Can you work these out from the model? Positions are in its coordinate system, mm. A direction names the side the tool comes from. Coordinates: 2 decimals unless noted, no trailing zeros. Order: outer loops, then holes, each group sorted by start corner. A loop starts at its lowest first (then second) coordinate and runs counter-clockwise, first axis right, second up.
```python
from build123d import *

# Parameters (mm, degrees)
SKETCH1_R           = 1.5
SKETCH1_R_2         = 3
BOSS_EXTRUDE1_DEPTH = 4
BOSS_EXTRUDE2_START = 4
SKETCH1_4_R         = 1.5
SKETCH1_4_R_2       = 3
BOSS_EXTRUDE2_DEPTH = 4
FILLET1_R           = 6
FILLET2_R           = 6
FILLET3_R           = 3
FILLET4_R           = 10


with BuildPart() as part:
    # Sketch1 → Boss-Extrude1 (new body)
    with BuildSketch(Plane(origin=(0, 0, 0), x_dir=(1, 0, 0), z_dir=(0, 1, 0))):
        Polygon((-84.75, 12.5), (-84.75, -12.5), (-67.174137787, -12.5), (-42.636751346, -55), (84.75, -55), (84.75, -45), (49.90212315, -45), (31.138239402, -12.5), (84.75, -12.5), (84.75, 12.5), (31.138239402, 12.5), (49.90212315, 45), (84.75, 45), (84.75, 55), (-42.636751346, 55), (-67.174137787, 12.5), align=None)
        Polygon((26.519437248, 12.5), (6.519437248, 12.5), (-12.244446501, 45), (45.283320997, 45), align=None, mode=Mode.SUBTRACT)
        Polygon((45.283320997, -45), (-12.244446501, -45), (6.519437248, -12.5), (26.519437248, -12.5), align=None, mode=Mode.SUBTRACT)
        Polygon((1.900635095, 12.5), (-55.627132403, 12.5), (-36.863248654, 45), (-16.863248654, 45), align=None, mode=Mode.SUBTRACT)
        Polygon((-16.863248654, -45), (-36.863248654, -45), (-55.627132403, -12.5), (1.900635095, -12.5), align=None, mode=Mode.SUBTRACT)
        with Locations(Location((-80.25, -7.5, 0), (0, 0, 270))):
            Circle(SKETCH1_R, mode=Mode.SUBTRACT)
        with Locations(Location((-65.25, -7.5, 0), (0, 0, 270))):
            Circle(SKETCH1_R, mode=Mode.SUBTRACT)
        with Locations(Location((-59.75, 0, 0), (0, 0, 270))):
            Circle(SKETCH1_R, mode=Mode.SUBTRACT)
        with Locations(Location((-49.75, 0, 0), (0, 0, 270))):
            Circle(SKETCH1_R, mode=Mode.SUBTRACT)
        with Locations(Location((-39.75, 0, 0), (0, 0, 270))):
            Circle(SKETCH1_R, mode=Mode.SUBTRACT)
        with Locations(Location((-29.75, 0, 0), (0, 0, 270))):
            Circle(SKETCH1_R, mode=Mode.SUBTRACT)
        with Locations(Location((-19.75, 0, 0), (0, 0, 270))):
            Circle(SKETCH1_R, mode=Mode.SUBTRACT)
        with Locations(Location((-9.75, 0, 0), (0, 0, 270))):
            Circle(SKETCH1_R, mode=Mode.SUBTRACT)
        with Locations(Location((0.25, 0, 0), (0, 0, 270))):
            Circle(SKETCH1_R, mode=Mode.SUBTRACT)
        with Locations(Location((10.25, 0, 0), (0, 0, 270))):
            Circle(SKETCH1_R, mode=Mode.SUBTRACT)
        with Locations(Location((20.25, 0, 0), (0, 0, 270))):
            Circle(SKETCH1_R, mode=Mode.SUBTRACT)
        with Locations(Location((30.25, 0, 0), (0, 0, 270))):
            Circle(SKETCH1_R, mode=Mode.SUBTRACT)
        with Locations(Location((40.25, 0, 0), (0, 0, 270))):
            Circle(SKETCH1_R, mode=Mode.SUBTRACT)
        with Locations(Location((50.25, 0, 0), (0, 0, 270))):
            Circle(SKETCH1_R, mode=Mode.SUBTRACT)
        with Locations(Location((-72.75, 0, 0), (0, 0, 270))):
            Circle(SKETCH1_R_2, mode=Mode.SUBTRACT)
        with Locations(Location((-80.25, 7.5, 0), (0, 0, 270))):
            Circle(SKETCH1_R, mode=Mode.SUBTRACT)
        with Locations(Location((-65.25, 7.5, 0), (0, 0, 270))):
            Circle(SKETCH1_R, mode=Mode.SUBTRACT)
        with Locations(Location((50.25, -50, 0), (0, 0, 270))):
            Circle(SKETCH1_R, mode=Mode.SUBTRACT)
        with Locations(Location((-39.75, -50, 0), (0, 0, 270))):
            Circle(SKETCH1_R, mode=Mode.SUBTRACT)
        with Locations(Location((-29.75, -50, 0), (0, 0, 270))):
            Circle(SKETCH1_R, mode=Mode.SUBTRACT)
        with Locations(Location((-19.75, -50, 0), (0, 0, 270))):
            Circle(SKETCH1_R, mode=Mode.SUBTRACT)
        with Locations(Location((-9.75, -50, 0), (0, 0, 270))):
            Circle(SKETCH1_R, mode=Mode.SUBTRACT)
        with Locations(Location((0.25, -50, 0), (0, 0, 270))):
            Circle(SKETCH1_R, mode=Mode.SUBTRACT)
        with Locations(Location((10.25, -50, 0), (0, 0, 270))):
            Circle(SKETCH1_R, mode=Mode.SUBTRACT)
        with Locations(Location((20.25, -50, 0), (0, 0, 270))):
            Circle(SKETCH1_R, mode=Mode.SUBTRACT)
        with Locations(Location((30.25, -50, 0), (0, 0, 270))):
            Circle(SKETCH1_R, mode=Mode.SUBTRACT)
        with Locations(Location((40.25, -50, 0), (0, 0, 270))):
            Circle(SKETCH1_R, mode=Mode.SUBTRACT)
        with Locations(Location((50.25, 50, 0), (0, 0, 270))):
            Circle(SKETCH1_R, mode=Mode.SUBTRACT)
        with Locations(Location((-39.75, 50, 0), (0, 0, 270))):
            Circle(SKETCH1_R, mode=Mode.SUBTRACT)
        with Locations(Location((-29.75, 50, 0), (0, 0, 270))):
            Circle(SKETCH1_R, mode=Mode.SUBTRACT)
        with Locations(Location((-19.75, 50, 0), (0, 0, 270))):
            Circle(SKETCH1_R, mode=Mode.SUBTRACT)
        with Locations(Location((-9.75, 50, 0), (0, 0, 270))):
            Circle(SKETCH1_R, mode=Mode.SUBTRACT)
        with Locations(Location((0.25, 50, 0), (0, 0, 270))):
            Circle(SKETCH1_R, mode=Mode.SUBTRACT)
        with Locations(Location((10.25, 50, 0), (0, 0, 270))):
            Circle(SKETCH1_R, mode=Mode.SUBTRACT)
        with Locations(Location((20.25, 50, 0), (0, 0, 270))):
            Circle(SKETCH1_R, mode=Mode.SUBTRACT)
        with Locations(Location((30.25, 50, 0), (0, 0, 270))):
            Circle(SKETCH1_R, mode=Mode.SUBTRACT)
        with Locations(Location((40.25, 50, 0), (0, 0, 270))):
            Circle(SKETCH1_R, mode=Mode.SUBTRACT)
        with Locations(Location((80.25, -50, 0), (0, 0, 270))):
            Circle(SKETCH1_R, mode=Mode.SUBTRACT)
        with Locations(Location((60.25, -50, 0), (0, 0, 270))):
            Circle(SKETCH1_R, mode=Mode.SUBTRACT)
        with Locations(Location((70.25, -50, 0), (0, 0, 270))):
            Circle(SKETCH1_R, mode=Mode.SUBTRACT)
        with Locations(Location((80.25, 50, 0), (0, 0, 270))):
            Circle(SKETCH1_R, mode=Mode.SUBTRACT)
        with Locations(Location((60.25, 50, 0), (0, 0, 270))):
            Circle(SKETCH1_R, mode=Mode.SUBTRACT)
        with Locations(Location((70.25, 50, 0), (0, 0, 270))):
            Circle(SKETCH1_R, mode=Mode.SUBTRACT)
        with Locations(Location((80.25, 0, 0), (0, 0, 270))):
            Circle(SKETCH1_R, mode=Mode.SUBTRACT)
        with Locations(Location((60.25, 0, 0), (0, 0, 270))):
            Circle(SKETCH1_R, mode=Mode.SUBTRACT)
        with Locations(Location((70.25, 0, 0), (0, 0, 270))):
            Circle(SKETCH1_R, mode=Mode.SUBTRACT)
    extrude(amount=-BOSS_EXTRUDE1_DEPTH)

    # Sketch1_4 → Boss-Extrude2 (add)
    with BuildSketch(Plane(origin=(0, 0, 0), x_dir=(1, 0, 0), z_dir=(0, 1, 0)).offset(BOSS_EXTRUDE2_START)):
        Polygon((-84.75, 12.5), (-84.75, -12.5), (-67.174137787, -12.5), (-42.636751346, -55), (55.25, -55), (55.25, -45), (49.90212315, -45), (31.138239402, -12.5), (55.25, -12.5), (55.25, 12.5), (31.138239402, 12.5), (49.90212315, 45), (55.25, 45), (55.25, 55), (-42.636751346, 55), (-67.174137787, 12.5), align=None)
        Polygon((26.519437248, 12.5), (6.519437248, 12.5), (-12.244446501, 45), (45.283320997, 45), align=None, mode=Mode.SUBTRACT)
        Polygon((45.283320997, -45), (-12.244446501, -45), (6.519437248, -12.5), (26.519437248, -12.5), align=None, mode=Mode.SUBTRACT)
        Polygon((1.900635095, 12.5), (-55.627132403, 12.5), (-36.863248654, 45), (-16.863248654, 45), align=None, mode=Mode.SUBTRACT)
        Polygon((-16.863248654, -45), (-36.863248654, -45), (-55.627132403, -12.5), (1.900635095, -12.5), align=None, mode=Mode.SUBTRACT)
        with Locations((-80.25, -7.5)):
            Circle(SKETCH1_4_R, mode=Mode.SUBTRACT)
        with Locations((-65.25, -7.5)):
            Circle(SKETCH1_4_R, mode=Mode.SUBTRACT)
        with Locations((-59.75, 0)):
            Circle(SKETCH1_4_R, mode=Mode.SUBTRACT)
        with Locations((-49.75, 0)):
            Circle(SKETCH1_4_R, mode=Mode.SUBTRACT)
        with Locations((-39.75, 0)):
            Circle(SKETCH1_4_R, mode=Mode.SUBTRACT)
        with Locations((-29.75, 0)):
            Circle(SKETCH1_4_R, mode=Mode.SUBTRACT)
        with Locations((-19.75, 0)):
            Circle(SKETCH1_4_R, mode=Mode.SUBTRACT)
        with Locations((-9.75, 0)):
            Circle(SKETCH1_4_R, mode=Mode.SUBTRACT)
        with Locations((0.25, 0)):
            Circle(SKETCH1_4_R, mode=Mode.SUBTRACT)
        with Locations((10.25, 0)):
            Circle(SKETCH1_4_R, mode=Mode.SUBTRACT)
        with Locations((20.25, 0)):
            Circle(SKETCH1_4_R, mode=Mode.SUBTRACT)
        with Locations((30.25, 0)):
            Circle(SKETCH1_4_R, mode=Mode.SUBTRACT)
        with Locations((40.25, 0)):
            Circle(SKETCH1_4_R, mode=Mode.SUBTRACT)
        with Locations((50.25, 0)):
            Circle(SKETCH1_4_R, mode=Mode.SUBTRACT)
        with Locations((-72.75, 0)):
            Circle(SKETCH1_4_R_2, mode=Mode.SUBTRACT)
        with Locations((-80.25, 7.5)):
            Circle(SKETCH1_4_R, mode=Mode.SUBTRACT)
        with Locations((-65.25, 7.5)):
            Circle(SKETCH1_4_R, mode=Mode.SUBTRACT)
        with Locations((50.25, -50)):
            Circle(SKETCH1_4_R, mode=Mode.SUBTRACT)
        with Locations((-39.75, -50)):
            Circle(SKETCH1_4_R, mode=Mode.SUBTRACT)
        with Locations((-29.75, -50)):
            Circle(SKETCH1_4_R, mode=Mode.SUBTRACT)
        with Locations((-19.75, -50)):
            Circle(SKETCH1_4_R, mode=Mode.SUBTRACT)
        with Locations((-9.75, -50)):
            Circle(SKETCH1_4_R, mode=Mode.SUBTRACT)
        with Locations((0.25, -50)):
            Circle(SKETCH1_4_R, mode=Mode.SUBTRACT)
        with Locations((10.25, -50)):
            Circle(SKETCH1_4_R, mode=Mode.SUBTRACT)
        with Locations((20.25, -50)):
            Circle(SKETCH1_4_R, mode=Mode.SUBTRACT)
        with Locations((30.25, -50)):
            Circle(SKETCH1_4_R, mode=Mode.SUBTRACT)
        with Locations((40.25, -50)):
            Circle(SKETCH1_4_R, mode=Mode.SUBTRACT)
        with Locations((50.25, 50)):
            Circle(SKETCH1_4_R, mode=Mode.SUBTRACT)
        with Locations((-39.75, 50)):
            Circle(SKETCH1_4_R, mode=Mode.SUBTRACT)
        with Locations((-29.75, 50)):
            Circle(SKETCH1_4_R, mode=Mode.SUBTRACT)
        with Locations((-19.75, 50)):
            Circle(SKETCH1_4_R, mode=Mode.SUBTRACT)
        with Locations((-9.75, 50)):
            Circle(SKETCH1_4_R, mode=Mode.SUBTRACT)
        with Locations((0.25, 50)):
            Circle(SKETCH1_4_R, mode=Mode.SUBTRACT)
        with Locations((10.25, 50)):
            Circle(SKETCH1_4_R, mode=Mode.SUBTRACT)
        with Locations((20.25, 50)):
            Circle(SKETCH1_4_R, mode=Mode.SUBTRACT)
        with Locations((30.25, 50)):
            Circle(SKETCH1_4_R, mode=Mode.SUBTRACT)
        with Locations((40.25, 50)):
            Circle(SKETCH1_4_R, mode=Mode.SUBTRACT)
    extrude(amount=-BOSS_EXTRUDE2_DEPTH)

    # Fillet1
    fillet1_edges = [part.edges().sort_by_distance(p)[0] for p in [
        (-84.75, 0, 12.5),
        (-84.75, 0, -12.5),
    ]]
    fillet(fillet1_edges, radius=FILLET1_R)

    # Fillet2
    fillet2_edges = [part.edges().sort_by_distance(p)[0] for p in [
        (-16.863248654, 0, -45),
        (-36.863248654, 0, -45),
        (49.90212315, 0, 45),
        (-67.174137787, 0, 12.5),
        (-67.174137787, 0, -12.5),
        (49.90212315, 0, -45),
        (26.519437248, 0, -12.5),
        (6.519437248, 0, -12.5),
        (-36.863248654, 0, 45),
        (-16.863248654, 0, 45),
        (26.519437248, 0, 12.5),
        (6.519437248, 0, 12.5),
    ]]
    fillet(fillet2_edges, radius=FILLET2_R)

    # Fillet3
    fillet3_edges = [part.edges().sort_by_distance(p)[0] for p in [
        (-55.627132403, 0, -12.5),
        (1.900635095, 0, -12.5),
        (31.138239402, 0, 12.5),
        (31.138239402, 0, -12.5),
        (45.283320997, 0, -45),
        (-12.244446501, 0, -45),
        (1.900635095, 0, 12.5),
        (-55.627132403, 0, 12.5),
        (-12.244446501, 0, 45),
        (45.283320997, 0, 45),
    ]]
    fillet(fillet3_edges, radius=FILLET3_R)

    # Fillet4
    fillet4_edges = [part.edges().sort_by_distance(p)[0] for p in [
        (-42.636751346, 0, 55),
        (-42.636751346, 0, -55),
    ]]
    fillet(fillet4_edges, radius=FILLET4_R)


solid = part.part
```
1. I'm going to push flat-ended pins straight in: pin 1 (2.5 mm diameter, centred on x = 63.5, y = 1, fed in from -Z); pin 2 (3 mm diameter, centred on x = 65.5, z = 51, fed in from +Y); pin 3 (2 mm diameter, centred on x = -56.5, y = 2.5, fed in from -Z). Where does each tip first touch, or does it pass through?
Completed:
pin 1: stops at z = -55
pin 2: stops at y = 0
pin 3: stops at z = -32.72
2. Please list where these lines run through material, in increasing order: probe 1 along Z at (x, y) = (10.25, 0); probe 2 along X at (y, z) = (-2.25, -7.5); probe 3 along X at (y, z) = (1, -22.5).
Completed:
probe 1: z = -55 to -51.5, -48.5 to -45, -12.5 to -1.5, 1.5 to 12.5, 45 to 48.5, 51.5 to 55
probe 2: x = -84.67 to -81.75, -78.75 to -66.75, -63.75 to 84.75
probe 3: x = -61.4 to -49.85, -3.87 to 0.75, 32.29 to 36.91
3. Thinking about a two-plate mould opening in Z: for faces 1 (the flat face through (-1, -4, 11)), 2 (the flat face through (-75, 0, 12.5)), 3 (the flat face through (-2.328, 0.056, -27.825)), which applies, pulls with the +Z half, pulls with the -Z half, needs draft (parallel to the pull), parting line crosses it, or undercut?
Completed:
face 1: needs draft
face 2: pulls with the +Z half
face 3: undercut
4. Imagine slicing it at B-B on y = -2.5. Give the number of separate pieces and of enclosed holes in the cut face, then the cut area to 3 significant figures.
Completed:
separate pieces: 1
enclosed holes: 50
area: 7,910 mm2
5. Imagine slicing it at A-A on x = 73.5. Please give me the cut outline in (y, z).
Completed:
outline: (-4, -55) - (0, -55) - (0, -45) - (-4, -45) - close; (-4, -12.5) - (0, -12.5) - (0, 12.5) - (-4, 12.5) - close; (-4, 45) - (0, 45) - (0, 55) - (-4, 55) - close
6. On a 3-axis mill with a long thin cutter (end or side, diameter ignored), from which of +Z, -Z, +X, -X, +Y, -Y can I reach the whole of each face in a straight line? I mean faces 4 (the flat face through (70, 0, 48)), 5 (the cylindrical face through (-83.039, -0.056, -10.696)), 6 (the flat face through (69, -2, -45)), 7 (the cylindrical face through (7.022, 0.056, -13.282)). Say none if no direction works.
Completed:
face 4: +Z, -Z, +X, +Y
face 5: -Z, -X, +Y, -Y
face 6: +X, +Y, -Y
face 7: +Y, -Y
